For this review, take the finished solid that the model builds, in its own axes (mm). A direction names the side the tool comes from. Round coordinates to 2 decimals unless told otherwise and drop trailing zeros. Order: outer loops, then holes, each group sorted by start corner. A loop starts at its lowest first (then second) coordinate and runs counter-clockwise, first axis right, second up. Notation, with made-up numbers: (46.5, 3) - (75.5, 3) arc R23 ccw to (75.5, 15) - close; hole circle Ø6 at (-2, 67). An arc over 180 degrees is marked (long way). Write each question's results on one line, items separated by ' | '. Start each with the question number.
(1) For faces 3 (the cylindrical face through (-15, 11.2, 7.4)), 4 (the flat face through (-13, 15, 4)), 5 (the flat face through (-12.5, 8, 8)), 6 (the cylindrical face through (9.885, 10.14, 6.749)), 7 (the flat face through (-3, 8, 0)), list the 3-axis set-ups (+Z, -Z, +X, -X, +Y, -Y) from which the entire face can be reached by the end or side of a thin tool; tool diameter is ignored.
(2) Take a section at A-A, the plane z = 7.5. Give the boundary of the cut face in (x, y), plus the area to 3 significant figures.
(3) For L1, parallel to X at y = 12.75, z = 7.5; L2, parallel to X at y = 6, z = 8; L3, parallel to Z at x = -12.5, y = 11.75, list the stretches that pass through material, from the lowest coordinate up. Write a range as from..to.
(4) Take a section at D-D, the plane x = -9. Give the boundary of the cut face in (y, z).
(5) Take a section at C-C, the plane y = 11.75. Give the boundary of the cut face in (x, z).
(6) Take a section at B-B, the plane y = 9.25. Give the boundary of the cut face in (x, z), plus the area to 3 significant figures.
(7) Insertion check: pin 1 Ø1 at (y, z) = (6, 13.5) entering from -X; pin 2 Ø2 at (x, z) = (6.5, 7) entering from -Y; pin 3 Ø1.2 at (x, z) = (-11.5, 7) entering from +Y. Each pin has a flat end and moves straight along its axis. Give the tip position at first contact, or say it passes through.
(8) Draft analysis for pull direction X (two halves, no side actions). For faces 1 (the flat face through (7, 0, 11)), 2 (the cylindrical face through (14.654, 9.86, 5.247)), state which applies: pulls with the +X half, pulls with the -X half, needs draft (parallel to the pull), parting line crosses it, or undercut.
```python
from build123d import *

# Parameters (mm, degrees)
CROQUIS1_R                = 7.5
SALIENTE_EXTRUIR1_DEPTH   = 20
SALIENTE_EXTRUIR1_2_DEPTH = 20
CROQUIS2_W                = 15
CROQUIS2_H                = 5
CORTAR_EXTRUIR1_DEPTH     = 20
CROQUIS3_W                = 15
CROQUIS3_H                = 5
CORTAR_EXTRUIR2_DEPTH     = 20
CROQUIS4_R                = 2.5
CORTAR_EXTRUIR3_DEPTH     = 20
CROQUIS5_R                = 2.5
CORTAR_EXTRUIR4_DEPTH     = 20
CROQUIS6_W                = 20
CROQUIS6_H                = 2.5
EXTRUIR_L_MINA1_DEPTH     = 15


with BuildPart() as part:
    # Croquis1 → Saliente-Extruir1 (new body)
    with BuildSketch(Plane(origin=(0, 0, 0), x_dir=(1, 0, 0), z_dir=(0, 1, 0))):
        with Locations((7.5, -7.5)):
            Circle(CROQUIS1_R)
    extrude(amount=SALIENTE_EXTRUIR1_DEPTH)

    # Croquis5 → Cortar-Extruir4 (cut)
    with BuildSketch(Plane(origin=(0, 20, 0), x_dir=(1, 0, 0), z_dir=(0, 1, 0))):
        with Locations((7.5, -7.5)):
            Circle(CROQUIS5_R)
    extrude(amount=-CORTAR_EXTRUIR4_DEPTH, mode=Mode.SUBTRACT)



with BuildPart() as body_2:
    # Croquis1 → Saliente-Extruir1 2 (new body)
    with BuildSketch(Plane(origin=(0, 0, 0), x_dir=(1, 0, 0), z_dir=(0, 1, 0))):
        with Locations((-12.5, -7.5)):
            Circle(CROQUIS1_R)
    extrude(amount=SALIENTE_EXTRUIR1_2_DEPTH)

    # Croquis2 → Cortar-Extruir1 (cut)
    with BuildSketch(Plane.XY.offset(15)):
        with Locations((-12.5, 2.5)):
            Rectangle(CROQUIS2_W, CROQUIS2_H)
    extrude(amount=-CORTAR_EXTRUIR1_DEPTH, mode=Mode.SUBTRACT)

    # Croquis3 → Cortar-Extruir2 (cut)
    with BuildSketch(Plane.XY.offset(15)):
        with Locations((-12.5, 17.5)):
            Rectangle(CROQUIS3_W, CROQUIS3_H)
    extrude(amount=-CORTAR_EXTRUIR2_DEPTH, mode=Mode.SUBTRACT)

    # Croquis4 → Cortar-Extruir3 (cut)
    with BuildSketch(Plane(origin=(0, 15, 0), x_dir=(1, 0, 0), z_dir=(0, 1, 0))):
        with Locations((-12.5, -7.5)):
            Circle(CROQUIS4_R)
    extrude(amount=-CORTAR_EXTRUIR3_DEPTH, mode=Mode.SUBTRACT)


with BuildPart() as part_1:
    add(part.part)

    add(body_2.part)  # Extruir-L_mina1 merges body 2
    # Croquis6 → Extruir-L_mina1 (add)
    with BuildSketch(Plane.XY.offset(15)):
        with Locations((-2.5, 6.25)):
            Rectangle(CROQUIS6_W, CROQUIS6_H)
        with Locations((-2.5, 8.75)):
            Rectangle(CROQUIS6_W, CROQUIS6_H)
    extrude(amount=-EXTRUIR_L_MINA1_DEPTH)


solid = part_1.part
```
Results below:
1) face 3: +Y | face 4: +Z, -Z, -X, +Y | face 5: +Y, -Y | face 6: none | face 7: -Z, +X, -X, +Y, -Y
2) outline: (-20, 5) - (-15, 5) - (-15, 15) - (-20, 15) - close; (-12.5, 5) - (0, 5) - (0, 0) - (5, 0) - (5, 5) - (7.5, 5) - (7.5, 10) - (5, 10) - (5, 20) - (0, 20) - (0, 10) - (-5, 10) - (-5, 15) - (-10, 15) - (-10, 10) - (-12.5, 10) - close; (10, 0) - (15, 0) - (15, 20) - (10, 20) - close | area: 350 mm^2
3) L1: x = -20..-15, -10..-5, 0..5, 10..15 | L2: x = -19.98..-14.95, -12.5..7.5, 9.95..14.98 | L3: z = 0..5, 10..15
4) outline: (5, 0) - (10, 0) - (10, 0.87) - (15, 0.87) - (15, 14.13) - (10, 14.13) - (10, 15) - (5, 15) - close
5) outline: circle Ø15 at (-12.5, 7.5); circle Ø15 at (7.5, 7.5); hole circle Ø5 at (-12.5, 7.5); hole circle Ø5 at (7.5, 7.5)
6) outline: (-12.5, 0) - (7.5, 0) arc R7.5 ccw to (7.5, 15) - (-12.5, 15) arc R7.5 ccw to start; hole (-12.5, 5) - (-12.5, 10) arc R2.5 ccw to start; hole (7.5, 5) arc R2.5 ccw to (7.5, 10) - close | area: 457 mm^2
7) pin 1: stops at x = -17.6 | pin 2: stops at y = 5 | pin 3: stops at y = 10
8) face 1: needs draft | face 2: undercut
